```python
from build123d import *

# Parameters (mm, degrees)
SKETCH2_W           = 31.75
SKETCH2_H           = 63.5
BOSS_EXTRUDE1_DEPTH = 3.175
SKETCH3_R           = 2.200000045
CUT_EXTRUDE1_DEPTH  = 4.175
BOSS_EXTRUDE2_START = -3.175
SKETCH4_W           = 3.175
SKETCH4_H           = 63.5
BOSS_EXTRUDE2_DEPTH = 19.05
BOSS_EXTRUDE3_DEPTH = 3.175
SKETCH6_R           = 1.700000029
CUT_EXTRUDE2_DEPTH  = 4.175


with BuildPart() as part:
    # Sketch2 → Boss-Extrude1 (new body)
    with BuildSketch(Plane.XY):
        with Locations((15.875, 31.75)):
            Rectangle(SKETCH2_W, SKETCH2_H)
    extrude(amount=BOSS_EXTRUDE1_DEPTH)

    # Sketch3 → Cut-Extrude1 (cut, through all)
    with BuildSketch(Plane.XY.offset(3.175)):
        with Locations((14.049999967, 9.827000031)):
            Circle(SKETCH3_R)
        with Locations((24.050000033, 9.827000031)):
            Circle(SKETCH3_R)
        with Locations((14.049999967, 58.427000113)):
            Circle(SKETCH3_R)
        with Locations((24.050000033, 58.427000113)):
            Circle(SKETCH3_R)
        Polygon((8.923000061, 54.704000066), (18.55, 54.704000066), (18.55, 61.308000066), (19.55, 61.308000066), (19.55, 54.704000066), (29.176999939, 54.704000066), (29.176999939, 13.550000078), (19.55, 13.550000078), (19.55, 6.946000078), (18.55, 6.946000078), (18.55, 13.550000078), (8.923000061, 13.550000078), align=None)
    extrude(amount=-CUT_EXTRUDE1_DEPTH, mode=Mode.SUBTRACT)

    # Sketch4 → Boss-Extrude2 (add)
    with BuildSketch(Plane.XY.offset(3.175).offset(BOSS_EXTRUDE2_START)):
        with Locations((1.5875, 31.75)):
            Rectangle(SKETCH4_W, SKETCH4_H)
    extrude(amount=-BOSS_EXTRUDE2_DEPTH)

    # Sketch5 → Boss-Extrude3 (add)
    with BuildSketch(Plane.XZ):
        Polygon((0, 3.175), (31.75, 3.175), (31.75, 0), (3.175, -19.05), (0, -19.05), align=None)
    extrude(amount=BOSS_EXTRUDE3_DEPTH)

    # Sketch6 → Cut-Extrude2 (cut, through all)
    with BuildSketch(Plane(origin=(3.175, 0, 0), x_dir=(0, 0, -1), z_dir=(1, 0, 0))):
        with Locations((3.175, 57.15)):
            Circle(SKETCH6_R)
        with Locations((3.175, 6.35)):
            Circle(SKETCH6_R)
        with Locations((15.875, 57.15)):
            Circle(SKETCH6_R)
        with Locations((15.875, 6.35)):
            Circle(SKETCH6_R)
    extrude(amount=-CUT_EXTRUDE2_DEPTH, mode=Mode.SUBTRACT)


solid = part.part
```
Here's how the part is built. I have some questions about the finished solid (model axes, mm). A direction names the side the tool comes from. Give positions to 0.01 mm unless a question says otherwise; leave off trailing zeros. Write each loop counter-clockwise with the first axis right and the second up, starting at its lowest first coordinate (ties: lowest second). Pieces come first, ordered by that corner, then holes.
(1) If I drill on L1, parallel to Y at x = 14.05, z = 2 (3 decimals); L2, parallel to Y at x = 3, z = -3 (3 decimals); L3, parallel to Z at x = 2, y = 57 (3 decimals), over which ranges is the centre line in solid material (lowest first)?
Output values:
L1: y = -3.175 to 7.627, 12.027 to 13.55, 54.704 to 56.227, 60.627 to 63.5
L2: y = -3.175 to 4.659, 8.041 to 55.459, 58.841 to 63.5
L3: z = -19.05 to -17.568, -14.182 to -4.868, -1.482 to 3.175
(2) Imagine slicing it at A-A, the plane x = 14.05. Write out the boundary of the cut face in (y, z) (3 decimals), and give its area (3 significant figures).
Output values:
outline: (-3.175, -11.8) - (0, -11.8) - (0, 0) - (7.627, 0) - (7.627, 3.175) - (-3.175, 3.175) - close; (12.027, 0) - (13.55, 0) - (13.55, 3.175) - (12.027, 3.175) - close; (54.704, 0) - (56.227, 0) - (56.227, 3.175) - (54.704, 3.175) - close; (60.627, 0) - (63.5, 0) - (63.5, 3.175) - (60.627, 3.175) - close
area: 90.6 mm2
(3) Thinking about a two-plate mould opening in X: for faces 4 (the face through (31.75, 31, 2)), 5 (the face through (15.233, 60.282, 1.61)), 6 (the face through (8, 32, 0)), which applies, pulls with the +X half, pulls with the -X half, needs draft (parallel to the pull), parting line crosses it, or undercut?
Output values:
face 4: pulls with the +X half
face 5: undercut
face 6: needs draft
(4) Imagine slicing it at C-C, the plane y = 57.15. Write out the boundary of the cut face in (x, z) (3 decimals), and give its area (3 significant figures).
Output values:
outline: (0, -19.05) - (3.175, -19.05) - (3.175, -17.575) - (0, -17.575) - close; (0, -14.175) - (3.175, -14.175) - (3.175, -4.875) - (0, -4.875) - close; (0, -1.475) - (3.175, -1.475) - (3.175, 0) - (12.259, 0) - (12.259, 3.175) - (0, 3.175) - close; (15.841, 0) - (18.55, 0) - (18.55, 3.175) - (15.841, 3.175) - close; (19.55, 0) - (22.259, 0) - (22.259, 3.175) - (19.55, 3.175) - close; (25.841, 0) - (31.75, 0) - (31.75, 3.175) - (25.841, 3.175) - close
area: 114 mm2
(5) On a 3-axis mill with a long thin cutter (end or side, diameter ignored), from which of +Z, -Z, +X, -X, +Y, -Y can I reach the whole of each face in a straight line? I mean faces 1 (the face through (24, 54.704, 2)), 2 (the face through (11, 0, -5)), 3 (the face through (10, 63.5, 1)). Say none if no direction works.
Output values:
face 1: +Z, -Z
face 2: -Z, +X, +Y
face 3: +Z, -Z, +X, -X, +Y
(6) Imagine slicing it at B-B, the plane y = 37.5. Write out the boundary of the cut face in (x, z) (3 decimals), and give its area (3 significant figures).
Output values:
outline: (0, -19.05) - (3.175, -19.05) - (3.175, 0) - (8.923, 0) - (8.923, 3.175) - (0, 3.175) - close; (29.177, 0) - (31.75, 0) - (31.75, 3.175) - (29.177, 3.175) - close
area: 97.0 mm2
(7) Imagine slicing it at D-D, the plane z = -12. Write out the boundary of the cut face in (x, y) (3 decimals), and give its area (3 significant figures).
Output values:
outline: (0, -3.175) - (13.75, -3.175) - (13.75, 0) - (3.175, 0) - (3.175, 63.5) - (0, 63.5) - close
area: 245 mm2
(8) Will these pins go through, and if not, where does the flat tip stop? pin 1 (5.5 mm diameter, centred on y = 57.15, z = -15.875, fed in from -X); pin 2 (6 mm diameter, centred on y = 51.5, z = -5, fed in from +X) (3 decimals); pin 3 (12 mm diameter, centred on x = 22.5, z = -10.5, fed in from +Y); pin 4 (8.5 mm diameter, centred on x = 13, y = 31, fed in from -Z).
Output values:
pin 1: stops at x = 0
pin 2: stops at x = 3.175
pin 3: stops at y = 0
pin 4: stops at z = 0
